Geometry: final body of the model. Coordinates: model frame, mm. A direction names the side the tool comes from. Give positions to 0.01 mm unless a question says otherwise; leave off trailing zeros. Loops run counter-clockwise (first coordinate to the right, second up) from the corner with the lowest first, then second, coordinate; pieces in that order, holes last. Notation, with made-up numbers: M 32.5,-5 L 86.5,-5 A25 cw 86.5,17 Z; hole C 31,84 d2. An arc over 180 degrees is marked long. Put each result on its own line as item: value.
```python
from build123d import *

# Parameters (mm, degrees)
BOSS_EXTRUDE1_DEPTH      = 38.1
BOSS_EXTRUDE2_DEPTH      = 38.1
BOSS_EXTRUDE2_DEPTH_BACK = 38.1
SKETCH3_R                = 10.16
CUT_EXTRUDE1_DEPTH       = 151.837563707


with BuildPart() as part:
    # Sketch1 → Boss-Extrude1 (new body)
    with BuildSketch(Plane(origin=(0, 0, 0), x_dir=(1, 0, 0), z_dir=(0, 1, 0))):
        with BuildLine():
            Line((50.8, 63.5), (0, 63.5))
            ThreePointArc((0, 63.5), (-35.921024484, 48.621024484), (-50.8, 12.7))
            Line((-50.8, 12.7), (-50.8, -12.7))
            ThreePointArc((-50.8, -12.7), (-35.921024484, -48.621024484), (0, -63.5))
            Line((0, -63.5), (50.8, -63.5))
            Line((50.8, -63.5), (50.8, 63.5))
        make_face()
    extrude(amount=BOSS_EXTRUDE1_DEPTH)

    # Sketch2 → Boss-Extrude2 (add, two sides: drawn at the far end of the back side and taken through both)
    with BuildSketch(Plane.XY.offset(-BOSS_EXTRUDE2_DEPTH_BACK)):
        with BuildLine():
            Line((50.8, 31.75), (88.9, 31.75))
            ThreePointArc((88.9, 31.75), (104.775, 15.875), (88.9, 0))
            Line((88.9, 0), (50.8, 0))
            Line((50.8, 0), (50.8, 31.75))
        make_face()
    extrude(amount=BOSS_EXTRUDE2_DEPTH + BOSS_EXTRUDE2_DEPTH_BACK)

    # Sketch3 → Cut-Extrude1 (cut, through all)
    with BuildSketch(Plane(origin=(0, 0, -38.1), x_dir=(-1, 0, 0), z_dir=(0, 0, -1))):
        with Locations((-88.9, 15.875)):
            Circle(SKETCH3_R)
    extrude(amount=-CUT_EXTRUDE1_DEPTH, mode=Mode.SUBTRACT)


solid = part.part
```
Item 1: Line query: probe 1 along Y at (x, z) = (88, 21); probe 2 along X at (y, z) = (16, 6.5); probe 3 along Y at (x, z) = (88.9, -11) (3 decimals). Output: solid intervals per line, ascending. Write a range as [from, to].
Output values:
probe 1: [0, 5.75], [26, 31.75]
probe 2: [-50.8, 78.74], [99.06, 104.77]
probe 3: [0, 5.715], [26.035, 31.75]
Item 2: Section D-D on y = 24. Output: boundary loops of the cut face in (x, z), then the cut area to 3 significant figures.
Output values:
outline: M -50.8,-12.7 A50.8 ccw 0,-63.5 L 50.8,-63.5 L 50.8,-38.1 L 82.8,-38.1 L 82.8,38.1 L 50.8,38.1 L 50.8,63.5 L 0,63.5 A50.8 ccw -50.8,12.7 Z; M 95,-38.1 L 102.54,-38.1 L 102.54,38.1 L 95,38.1 Z
area: 14,800 mm²
Item 3: Section A-A on z = -23. Output: boundary loops of the cut face in (x, y) (3 decimals).
Output values:
outline: M -49.745,0 L 88.9,0 A15.875 ccw 88.9,31.75 L 50.8,31.75 L 50.8,38.1 L -49.745,38.1 Z; hole C 88.9,15.875 d20.32
Item 4: Mould query, pull axis Y, two halves, no side actions, for faces 5 (the flat face through (-1, 38.1, -1)), 6 (the cylindrical face through (79.515, 11.984, -0.533)), 7 (the cylindrical face through (104.77, 16.22, -0.53)). Classes: pulls with the +Y half, pulls with the -Y half, needs draft (parallel to the pull), parting line crosses it, or undercut.
Output values:
face 5: pulls with the +Y half
face 6: undercut
face 7: parting line crosses it
Item 5: Section C-C on y = 35.5. Output: boundary loops of the cut face in (x, z).
Output values:
outline: M -50.8,-12.7 A50.8 ccw 0,-63.5 L 50.8,-63.5 L 50.8,63.5 L 0,63.5 A50.8 ccw -50.8,12.7 Z
Item 6: Section B-B on x = 84.5. Output: boundary loops of the cut face in (y, z).
Output values:
outline: M 0,-38.1 L 6.72,-38.1 L 6.72,38.1 L 0,38.1 Z; M 25.03,-38.1 L 31.75,-38.1 L 31.75,38.1 L 25.03,38.1 Z
Item 7: Set-up query: faces 1 (the flat face through (25, 19, 63.5)), 2 (the flat face through (72, 16, -38.1)), 3 (the flat face through (70, 31.75, -1)), 4 (the flat face through (72, 16, 38.1)). Return all of +Z, -Z, +X, -X, +Y, -Y with unobstructed straight access to the full face (end or side cutting, diameter ignored); none if empty.
Output values:
face 1: +Z, +X, -X, +Y, -Y
face 2: -Z, +X, +Y, -Y
face 3: +Z, -Z, +X, +Y
face 4: +Z, +X, +Y, -Y
Item 8: Pin query (flat end, axial travel): pin 1 Ø16 at (x, y) = (75, 21.5) entering from -Z; pin 2 Ø8 at (x, y) = (-16.5, 33.5) entering from -Z; pin 3 Ø5 at (y, z) = (26, 2) entering from +X. Return the tip coordinate at first contact, or that it passes through.
Output values:
pin 1: z = -38.1
pin 2: z = -61.94
pin 3: x = 102.82
